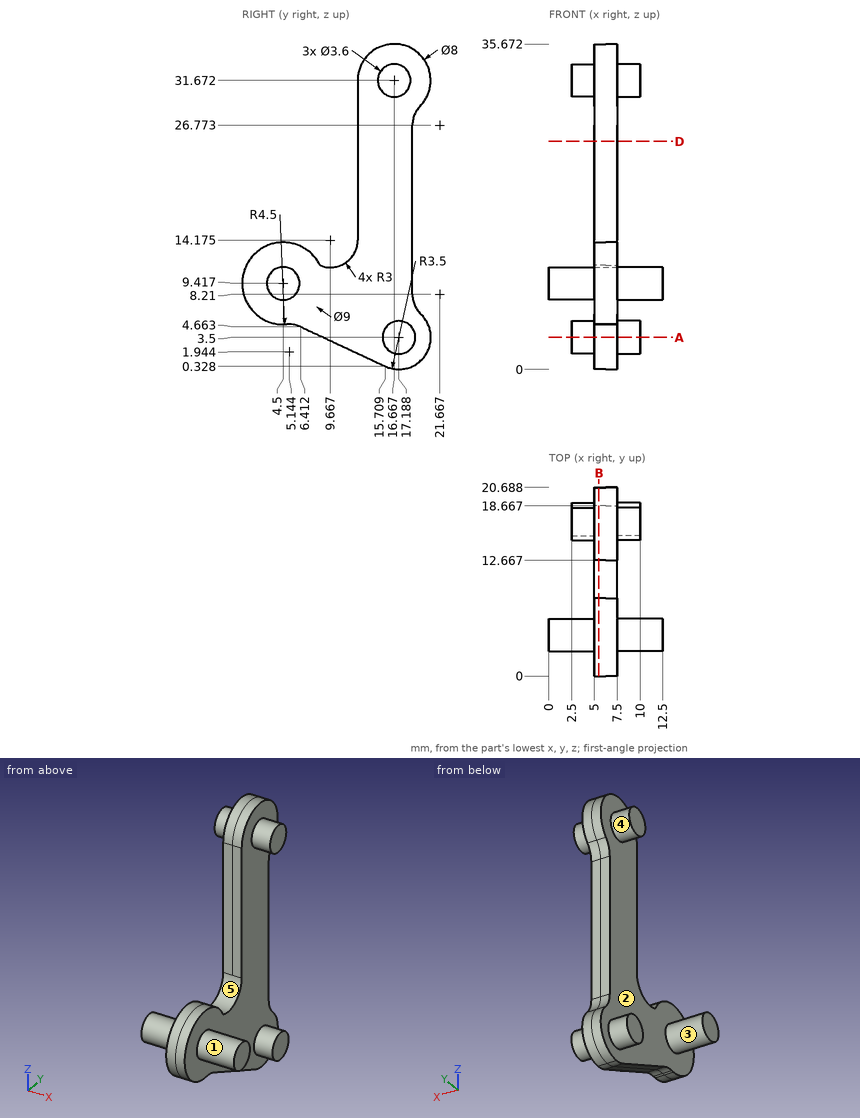
Geometry: see drawing. Coordinates: mm, zero at the bounding-box minimum. A direction names the side the tool comes from. Round coordinates to 2 decimals unless told otherwise and drop trailing zeros. Order: outer loops, then holes, each group sorted by start corner. A loop starts at its lowest first (then second) coordinate and runs counter-clockwise, first axis right, second up. Notation, with made-up numbers: (58.25, 49) - (111.25, 49) arc R7 ccw to (111.25, 61) - close; hole circle Ø3 at (3.5, -23). An arc over 180 degrees is marked (long way). One line per question, with ' | ' between items. Start each with the question number.
1) Ray query, probe 1 along X at (y, z) = (15.75, 27); probe 2 along Z at (x, y) = (5.5, 9.75) (1 decimal); probe 3 along Z at (x, y) = (6, 18.5) (1 decimal). Return the intervals inside material, ascending.
2) Cut plane A-A, the plane z = 3.5. Return the cut outline in (x, y).
3) Cut plane D-D, the plane z = 25. Return the cut outline in (x, y), then the cut area to 3 significant figures.
4) Pull-direction query (Z, two-part tool) for the marked faces 3, 4 and 5; classes: +Z half, -Z half, draft (parallel to the pull), parting line (faces both ways), or undercut.
5) Cut plane B-B, the plane x = 5.5. Return the cut outline in (y, z) (1 decimal), then the cut area to 3 significant figures.
6) Contact query for flat-ended pins moving along their axis: P1, Ø1.4, axis at x = 6, z = 19.5, coming from the -Y side; P2, Ø2, axis at x = 10.5, y = 12.5, coming from the +Z side; P3, Ø10, axis at y = 12, z = 31.5, coming from the +X side; P4, Ø1.8, axis at y = 18, z = 3, coming from the -X side. Output: stop coordinate, or through.
7) Set-up query: the marked faces 1 and 2. Return all of +Z, -Z, +X, -X, +Y, -Y with unobstructed straight access to the full face (end or side cutting, diameter ignored); none if empty.
Worked out:
1) probe 1: x = 5 to 7.5 | probe 2: z = 3.1 to 11.2 | probe 3: z = 0.3 to 35.2
2) outline: (2.5, 15.39) - (5, 15.39) - (5, 8.91) - (7.5, 8.91) - (7.5, 15.39) - (10, 15.39) - (10, 18.99) - (7.5, 18.99) - (7.5, 20.69) - (5, 20.69) - (5, 18.99) - (2.5, 18.99) - close
3) outline: (5, 12.67) - (7.5, 12.67) - (7.5, 18.67) - (5, 18.67) - close | area: 15.0 mm^2
4) face 3: parting line | face 4: undercut | face 5: +Z half
5) outline: (4.9, 4.9) arc R3 cw to (6.4, 4.7) - (15.7, 0.3) arc R3.5 ccw to (19.6, 6) arc R3 cw to (18.7, 8.2) - (18.7, 26.8) arc R3 cw to (19.5, 28.9) arc R4 ccw (long way) to (12.7, 31.7) - (12.7, 14.2) arc R3 cw to (8.5, 11.4) arc R4.5 ccw (long way) to start | area: 330 mm^2
6) P1: stops at y = 12.67 | P2: passes through | P3: stops at x = 10 | P4: stops at x = 2.5
7) face 1: +X | face 2: -X
